Source: three-view drawing plus pictorial views. Frame: mm from the lowest corner of the part. A direction names the side the tool comes from. Give positions to 0.01 mm unless a question says otherwise; leave off trailing zeros. Write each loop counter-clockwise with the first axis right and the second up, starting at its lowest first coordinate (ties: lowest second). Pieces come first, ordered by that corner, then holes. Notation, with made-up numbers: (-19, 38.5) -> (-1, 38.5) arc R24 ccw to (-1, 51.5) -> close; hole circle Ø1 at (47.5, -2). An arc over 180 degrees is marked (long way). Write item = value, one per line.
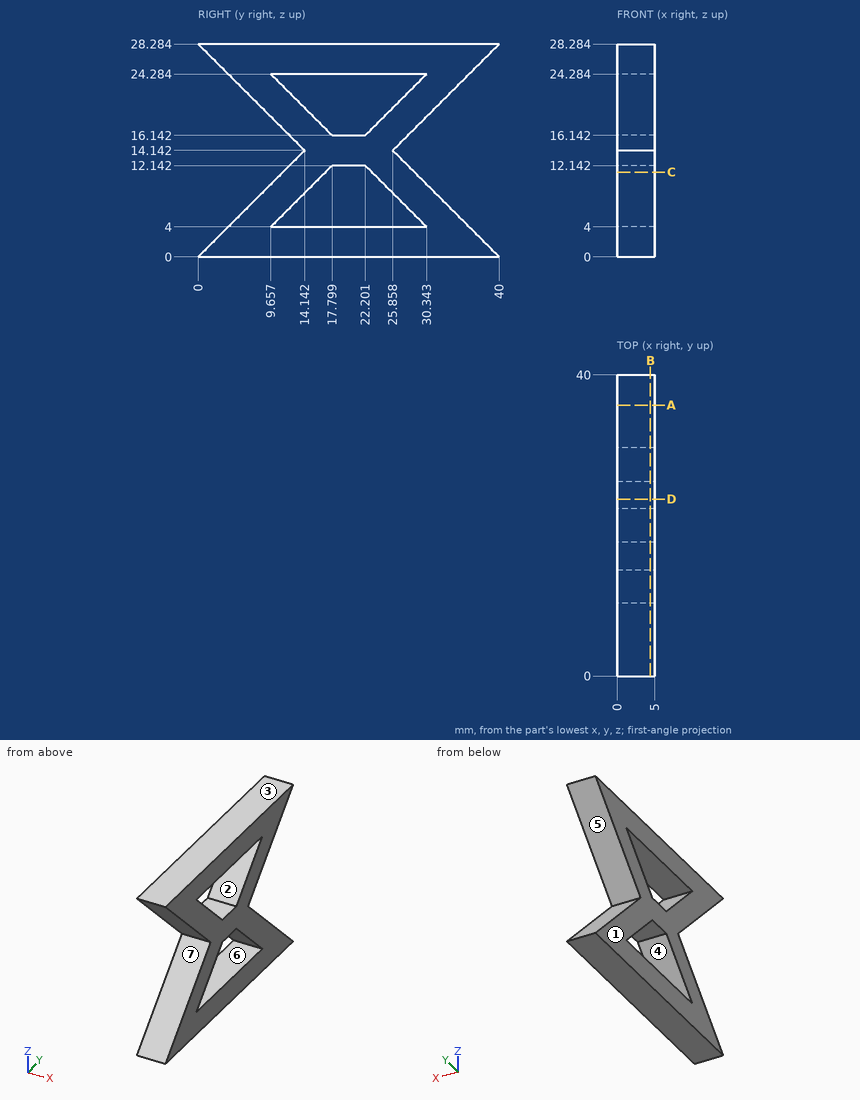
1) Cut plane D-D (y = 23.5). Return the cut outline in (x, z).
Computed:
outline = (0, 0) -> (5, 0) -> (5, 4) -> (0, 4) -> close; (0, 10.84) -> (5, 10.84) -> (5, 17.44) -> (0, 17.44) -> close; (0, 24.28) -> (5, 24.28) -> (5, 28.28) -> (0, 28.28) -> close
2) Cut plane B-B (x = 4.4). Return the cut outline in (y, z), then the cut area to 3 significant figures.
Computed:
outline = (0, 0) -> (40, 0) -> (25.86, 14.14) -> (40, 28.28) -> (0, 28.28) -> (14.14, 14.14) -> close; hole (9.66, 4) -> (30.34, 4) -> (22.2, 12.14) -> (17.8, 12.14) -> close; hole (9.66, 24.28) -> (17.8, 16.14) -> (22.2, 16.14) -> (30.34, 24.28) -> close
area = 527 mm²
3) Material intervals for L1, parallel to Z at x = 3.55, y = 21.5; L2, parallel to Z at x = 2.8, y = 25.5 (1 decimal); L3, parallel to Z at x = 3.85, y = 29 (1 decimal), sorted ascending.
Computed:
L1 = 0 to 4, 12.14 to 16.14, 24.28 to 28.28
L2 = 0 to 4, 8.8 to 19.4, 24.3 to 28.3
L3 = 0 to 4, 5.3 to 11, 17.3 to 22.9, 24.3 to 28.3
4) Cut plane A-A (y = 36). Return the cut outline in (x, z), then the cut area to 3 significant figures.
Computed:
outline = (0, 0) -> (5, 0) -> (5, 4) -> (0, 4) -> close; (0, 24.28) -> (5, 24.28) -> (5, 28.28) -> (0, 28.28) -> close
area = 40.0 mm²
5) Access query for the marked faces 5, 6 and 7. Directions: +Z, -Z, +X, -X, +Y, -Y. A direction counts if a zero-diameter tool reaches every point of the face in a straight line with its end or side. Return the directions, or none.
Computed:
face_5 = +X, -X, +Y
face_6 = +X, -X
face_7 = +X, -X, -Y
6) Draft query along Z for the marked faces 1, 2, 3 and 4. Return one class per face: pulls with the +Z half, pulls with the -Z half, needs draft (parallel to the pull), parting line crosses it, or undercut.
Computed:
face_1 = needs draft
face_2 = undercut
face_3 = pulls with the +Z half
face_4 = undercut
7) Contact query for flat-ended pins moving along their axis: pin 1 (1 mm diameter, centred on x = 0.5, z = 3, fed in from +Y); pin 2 (1.5 mm diameter, centred on x = 3, y = 24, fed in from -Z). Output: stop coordinate, or through.
Computed:
pin_1 = 37.5
pin_2 = 0
8) Cut plane C-C (z = 11.25). Return the cut outline in (x, y).
Computed:
outline = (0, 11.25) -> (5, 11.25) -> (5, 16.91) -> (0, 16.91) -> close; (0, 23.09) -> (5, 23.09) -> (5, 28.75) -> (0, 28.75) -> close
